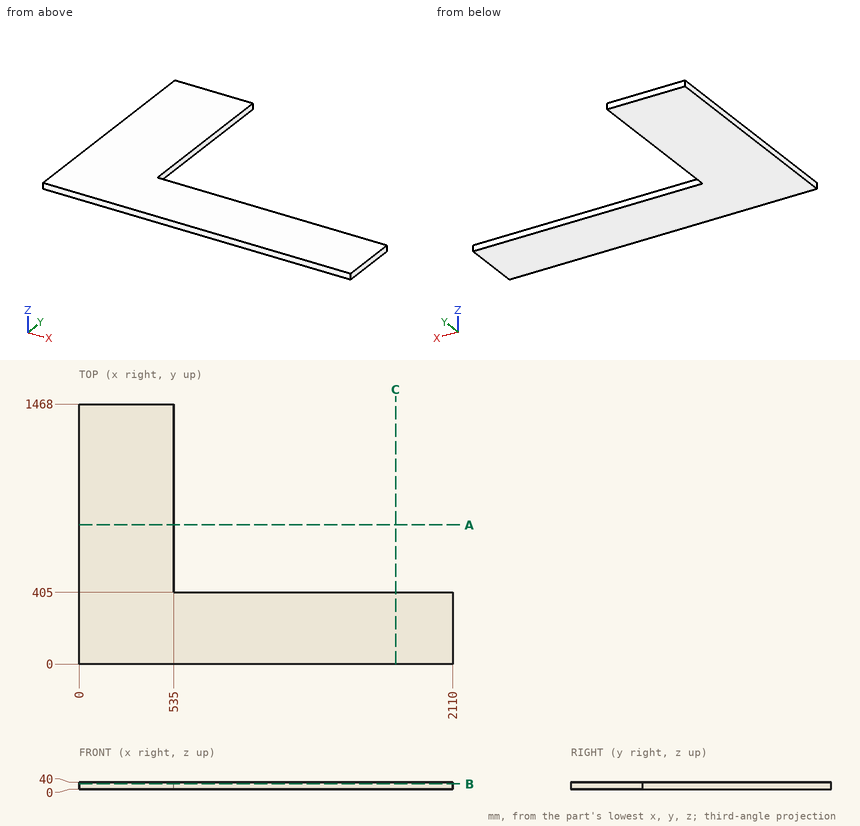
Verification items for this drawing (mm, ordinates from the low corner). Coordinates: 2 decimals unless noted, no trailing zeros. Loops run counter-clockwise (first coordinate to the right, second up) from the corner with the lowest first, then second, coordinate; pieces in that order, holes last. Notation, with made-up numbers: (25.25, 70.25) -> (57.25, 70.25) arc R23 cw to (57.25, 84.25) -> close; hole circle Ø6 at (34, -5). An arc over 180 degrees is marked (long way). Answer in a Markdown table with one row per item. Add a question column.
1. Section check C-C, the plane x = 1787. Enter the section's corners in (y, z), then the cut area to 3 significant figures.
2. Material ranges on probe 1 along Y at (x, z) = (1105.5, 7); probe 2 along X at (y, z) = (1029, 4), recorded low to high. Write a range as [from, to].
3. Depth check by flat-ended pin: P1, Ø2, axis at y = 793.5, z = 25, coming from the +X side; P2, Ø2, axis at x = 1166, z = 10.5, coming from the +Y side. Enter the tip coordinate at first touch or a pass-through.
4. Section check B-B, the plane z = 30. Enter the section's corners in (x, y).
5. Section check A-A, the plane y = 785.5. Enter the section's corners in (x, z), then the cut area to 3 significant figures.
Derived:
| question | item | result |
|---|---|---|
| 1 | outline | (0, 0) -> (405, 0) -> (405, 40) -> (0, 40) -> close |
| 1 | area | 16,200 mm² |
| 2 | probe 1 | y = [0, 405] |
| 2 | probe 2 | x = [0, 535] |
| 3 | P1 | stops at x = 535 |
| 3 | P2 | stops at y = 405 |
| 4 | outline | (0, 0) -> (2110, 0) -> (2110, 405) -> (535, 405) -> (535, 1468) -> (0, 1468) -> close |
| 5 | outline | (0, 0) -> (535, 0) -> (535, 40) -> (0, 40) -> close |
| 5 | area | 21,400 mm² |
